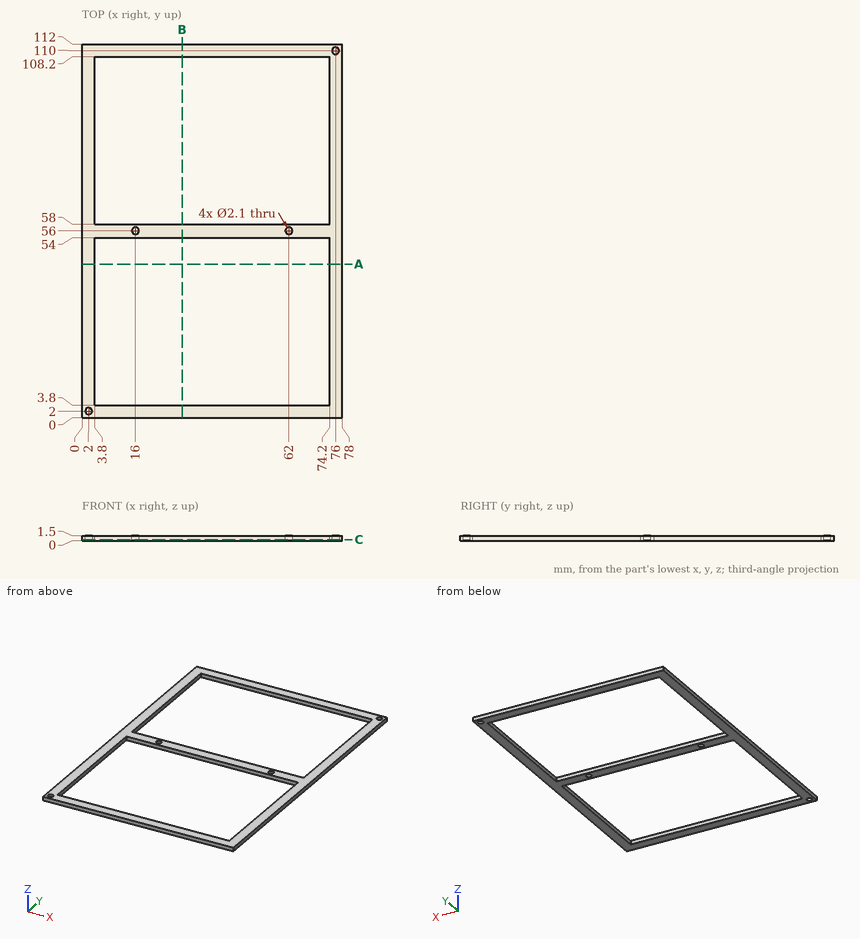
Can you work these out from the drawing? Everything is in mm from the part's minimum corner. Coordinates: 2 decimals unless noted, no trailing zeros. Order: outer loops, then holes, each group sorted by start corner. A loop starts at its lowest first (then second) coordinate and runs counter-clockwise, first axis right, second up. Notation, with made-up numbers: M -32.75,-29.75 L 22.25,-29.75 A21 cw 22.25,1.25 Z; hole C 36.25,16 d5. An arc over 180 degrees is marked long. Answer as CSV lines item,"result". Start each with the question number.
1. I need wall thicknesses on line 1 (Y direction, x = 62, z = 1); line 2 (Y direction, x = 33.5, z = 0.4); line 3 (X direction, y = 99, z = 0.9). Which ranges of each line are inside material? Lowest first, please. Write a range as [from, to].
2. I want a section at B-B, the plane x = 30. Write out the boundary of the cut face in (y, z).
3. I want a section at A-A, the plane y = 46. Write out the boundary of the cut face in (x, z), and give its area (3 significant figures).
4. I want a section at C-C, the plane z = 0.35. Write out the boundary of the cut face in (x, y), and give its area (3 significant figures).
Recorded:
1,line 1,"y = [0, 3.8], [54, 54.95], [57.05, 58], [108.2, 112]"
1,line 2,"y = [0, 3.8], [54, 58], [108.2, 112]"
1,line 3,"x = [0, 3.8], [74.2, 78]"
2,outline,"M 0,0 L 3.8,0 L 3.8,1.5 L 0,1.5 Z; M 54,0 L 58,0 L 58,1.5 L 54,1.5 Z; M 108.2,0 L 112,0 L 112,1.5 L 108.2,1.5 Z"
3,outline,"M 0,0 L 3.8,0 L 3.8,1.5 L 0,1.5 Z; M 74.2,0 L 78,0 L 78,1.5 L 74.2,1.5 Z"
3,area,"11.4 mm2"
4,outline,"M 0,0 L 78,0 L 78,112 L 0,112 Z; hole C 2,2 d2.1; hole M 3.8,3.8 L 74.2,3.8 L 74.2,54 L 3.8,54 Z; hole M 3.8,58 L 74.2,58 L 74.2,108.2 L 3.8,108.2 Z; hole C 16,56 d2.1; hole C 62,56 d2.1; hole C 76,110 d2.1"
4,area,"1,650 mm2"
